Source: CAD feature listing. Evaluate the final solid. Frame: model axes, mm. A direction names the side the tool comes from. Round coordinates to 2 decimals unless told otherwise and drop trailing zeros. Write each loop counter-clockwise with the first axis right and the second up, starting at its lowest first coordinate (ties: lowest second). Pieces come first, ordered by that corner, then holes. Notation, with made-up numbers: (61, 11) -> (71, 11) arc R30 cw to (71, 37) -> close; hole circle Ø5 at (-7.5, 24.25). An arc over 180 degrees is marked (long way). Put each result on its own line as item: value.
```python
from build123d import *

# Parameters (mm, degrees)
F0_R     = 21.2
F1_DEPTH = 17.1
F2_R     = 12.7
F3_DEPTH = 2
F5_R     = 2.15
F6_DEPTH = 25
F7_R     = 3.1
F8_DEPTH = 8.001


with BuildPart() as f1:
    # F0 (on Top) → F1 (new body)
    with BuildSketch(Plane.XY):
        with BuildLine():
            Line((-54.2, -26.2), (54.2, -26.2))
            Line((54.2, -26.2), (54.2, -18.2))
            Line((54.2, -18.2), (29.2, -18.2))
            Line((29.2, -18.2), (29.2, 0))
            ThreePointArc((29.2, 0), (0, 29.2), (-29.2, 0))
            Line((-29.2, 0), (-29.2, -18.2))
            Line((-29.2, -18.2), (-54.2, -18.2))
            Line((-54.2, -18.2), (-54.2, -26.2))
        make_face()
        Circle(F0_R, mode=Mode.SUBTRACT)
    extrude(amount=F1_DEPTH)

    # F2 (on face) → F3 (join)
    with BuildSketch(Plane(origin=(0, 0, 0), x_dir=(1, 0, 0), z_dir=(0, 0, -1))):
        with BuildLine():
            Line((-29.2, 18.2), (-29.2, 0))
            ThreePointArc((-29.2, 0), (0, -29.2), (29.2, 0))
            Line((29.2, 0), (29.2, 18.2))
            Line((29.2, 18.2), (54.2, 18.2))
            Line((54.2, 18.2), (54.2, 26.2))
            Line((54.2, 26.2), (-54.2, 26.2))
            Line((-54.2, 26.2), (-54.2, 18.2))
            Line((-54.2, 18.2), (-29.2, 18.2))
        make_face()
        Circle(F2_R, mode=Mode.SUBTRACT)
    extrude(amount=F3_DEPTH)

    # F5 (on face) → F6 (cut)
    with BuildSketch(Plane.XY):
        with Locations((11.327767, 13.988627)):
            Circle(F5_R)
        with Locations((13.988627, -11.327767)):
            Circle(F5_R)
        with Locations((-11.327767, -13.988627)):
            Circle(F5_R)
        with Locations((-13.988627, 11.327767)):
            Circle(F5_R)
    extrude(amount=-F6_DEPTH, mode=Mode.SUBTRACT)

    # F7 (on face) → F8 (cut, through all)
    with BuildSketch(Plane(origin=(0, -18.2, 0), x_dir=(-1, 0, 0), z_dir=(0, 1, 0))):
        with Locations((41.7, 7.55)):
            Circle(F7_R)
        with Locations((-41.7, 7.55)):
            Circle(F7_R)
    extrude(amount=-F8_DEPTH, mode=Mode.SUBTRACT)


solid = f1.part
```
Q1. Cut plane A-A on z = 7.55. Output: boundary loops of the cut face in (x, y).
Ans:
outline: (-54.2, -26.2) -> (-44.8, -26.2) -> (-44.8, -18.2) -> (-54.2, -18.2) -> close; (-38.6, -26.2) -> (38.6, -26.2) -> (38.6, -18.2) -> (29.2, -18.2) -> (29.2, 0) arc R29.2 ccw to (-29.2, 0) -> (-29.2, -18.2) -> (-38.6, -18.2) -> close; (44.8, -26.2) -> (54.2, -26.2) -> (54.2, -18.2) -> (44.8, -18.2) -> close; hole circle Ø42.4 at (0, 0)
Q2. Reachability of faces 4 (the cylindrical face through (19.583, -8.12, 8.43)), 5 (the flat face through (-29.2, -9, 8)), 6 (the cylindrical face through (-11.608, -11.857, -0.986)), 7 (the cylindrical face through (-0.642, 29.193, 7.684)), 8 (the flat face through (29.2, -9, 8)) from +Z, -Z, +X, -X, +Y, -Y: full face, straight path, thin tool, end or side. Return the list, or none.
Ans:
face 4: +Z
face 5: +Z, -Z, -X, +Y
face 6: +Z, -Z
face 7: +Z, -Z, +Y
face 8: +Z, -Z, +X, +Y
Q3. Draft query along Z for faces 1 (the flat face through (-54.2, -22, 8)), 2 (the cylindrical face through (38.836, -22.144, 6.363)), 3 (the flat face through (9.1, 9.1, 0)). Return one class per face: +Z half, -Z half, draft (parallel to the pull), parting line (faces both ways), or undercut.
Ans:
face 1: draft
face 2: undercut
face 3: +Z half
Q4. Pin query (flat end, axial travel): pin 1 (5 mm diameter, centred on x = -38.5, z = 9.5, fed in from +Y); pin 2 (6 mm diameter, centred on y = 12, z = 10, fed in from +X); pin 3 (9 mm diameter, centred on y = -9, z = 7, fed in from -X). Return the tip coordinate at first contact, or that it passes through.
Ans:
pin 1: stops at y = -18.2
pin 2: stops at x = 27.78
pin 3: stops at x = -29.2
Q5. Cut plane C-C on y = -6.5. Output: boundary loops of the cut face in (x, z), and give its area (3 significant figures).
Ans:
outline: (-29.2, -2) -> (-10.91, -2) -> (-10.91, 0) -> (-20.18, 0) -> (-20.18, 17.1) -> (-29.2, 17.1) -> close; (10.91, -2) -> (29.2, -2) -> (29.2, 17.1) -> (20.18, 17.1) -> (20.18, 0) -> (10.91, 0) -> close
area: 382 mm^2
Q6. Material intervals for line 1 (X direction, y = 0, z = -0.75); line 2 (Z direction, x = 41.7, y = -23.25); line 3 (Y direction, x = 30, z = 9.75), sorted ascending. Write a range as [from, to].
Ans:
line 1: x = [-29.2, -12.7], [12.7, 29.2]
line 2: z = [-2, 4.45], [10.65, 17.1]
line 3: y = [-26.2, -18.2]
Q7. Cut plane B-B on x = 0. Output: boundary loops of the cut face in (y, z), and give its area (3 significant figures).
Ans:
outline: (-26.2, -2) -> (-12.7, -2) -> (-12.7, 0) -> (-21.2, 0) -> (-21.2, 17.1) -> (-26.2, 17.1) -> close; (12.7, -2) -> (29.2, -2) -> (29.2, 17.1) -> (21.2, 17.1) -> (21.2, 0) -> (12.7, 0) -> close
area: 282 mm^2
Q8. Cut plane D-D on z = 15.75. Output: boundary loops of the cut face in (x, y).
Ans:
outline: (-54.2, -26.2) -> (54.2, -26.2) -> (54.2, -18.2) -> (29.2, -18.2) -> (29.2, 0) arc R29.2 ccw to (-29.2, 0) -> (-29.2, -18.2) -> (-54.2, -18.2) -> close; hole circle Ø42.4 at (0, 0)
